Answer from the drawing. Dimensions are ordinates in mm from the lowest x, y and z of the part. A direction names the side the tool comes from. Round coordinates to 2 decimals unless told otherwise and drop trailing zeros. Loops run counter-clockwise (first coordinate to the right, second up) from the corner with the lowest first, then second, coordinate; pieces in that order, holes last. Notation, with made-up numbers: M 0.25,33 L 30.25,33 A16 cw 30.25,59 Z; hole C -5,51.5 d5. An arc over 180 degrees is marked long. Answer as a JSON object with one key per item and string values.
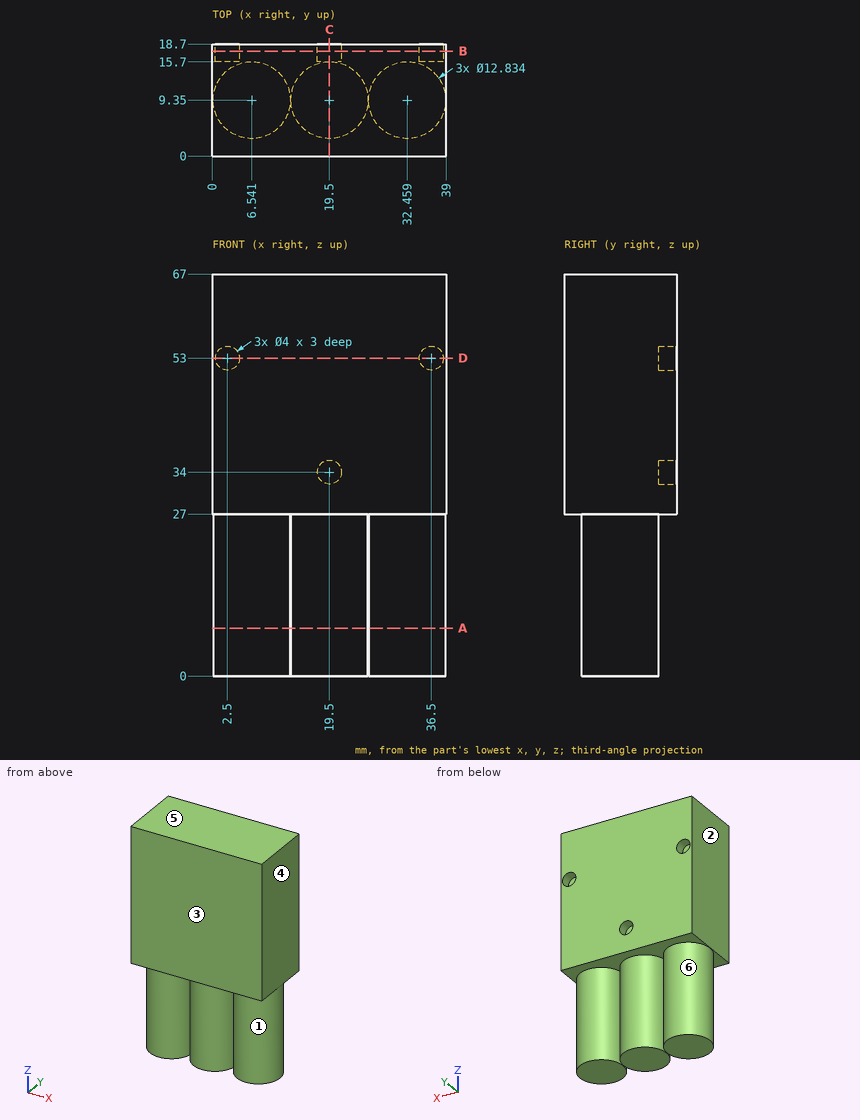
Item 1: Straight lines are drawn through the part: line 1 (Z direction, x = 36.5, y = 17.45); line 2 (X direction, y = 18, z = 34); line 3 (Z direction, x = 19.5, y = 16.8). For each, find the intervals that lie inside material, in ascending order.
Values follow:
{"line 1": "27 to 51, 55 to 67", "line 2": "0 to 17.5, 21.5 to 39", "line 3": "27 to 32, 36 to 67"}
Item 2: The part is cut by section B-B (y = 17.5). Give the vertices of the cut face in (x, z).
Values follow:
{"outline": "M 0,27 L 39,27 L 39,67 L 0,67 Z; hole C 2.5,53 d4; hole C 19.5,34 d4; hole C 36.5,53 d4"}
Item 3: Which of the six approach directions +Z, -Z, +X, -X, +Y, -Y give full straight-line access (tool end or side, diameter ignored) to the marked faces 5 and 6?
Values follow:
{"face 5": "+Z, +X, -X, +Y, -Y", "face 6": "-Z"}
Item 4: The part is cut by section C-C (x = 19.5). Give the vertices of the cut face in (y, z).
Values follow:
{"outline": "M 0,27 L 2.93,27 L 2.93,0 L 15.77,0 L 15.77,27 L 18.7,27 L 18.7,32 L 15.7,32 L 15.7,36 L 18.7,36 L 18.7,67 L 0,67 Z"}
Item 5: Flat-ended cylindrical pins translate along their axes: P1, Ø5, axis at y = 11.5, z = 50, coming from the -X side; P2, Ø3, axis at x = 2.5, z = 53, coming from the +Y side. Find the tip coordinate at first contact, or state that the pin passes through.
Values follow:
{"P1": "x = 0", "P2": "y = 15.7"}
Item 6: Determine the mould class of the marked faces 1, 2, 3 and 4 for opening direction X: released by +X, released by -X, zero draft, split by the parting line, or undercut.
Values follow:
{"face 1": "undercut", "face 2": "released by -X", "face 3": "zero draft", "face 4": "released by +X"}
Item 7: The part is cut by section A-A (z = 8). Give the number of separate pieces and of enclosed holes in the cut face, then the cut area to 3 significant figures.
Values follow:
{"separate pieces": "3", "enclosed holes": "0", "area": "388 mm^2"}
Item 8: The part is cut by section D-D (z = 53). Give the vertices of the cut face in (x, y), then the cut area to 3 significant figures.
Values follow:
{"outline": "M 0,0 L 39,0 L 39,18.7 L 38.5,18.7 L 38.5,15.7 L 34.5,15.7 L 34.5,18.7 L 4.5,18.7 L 4.5,15.7 L 0.5,15.7 L 0.5,18.7 L 0,18.7 Z", "area": "705 mm^2"}
